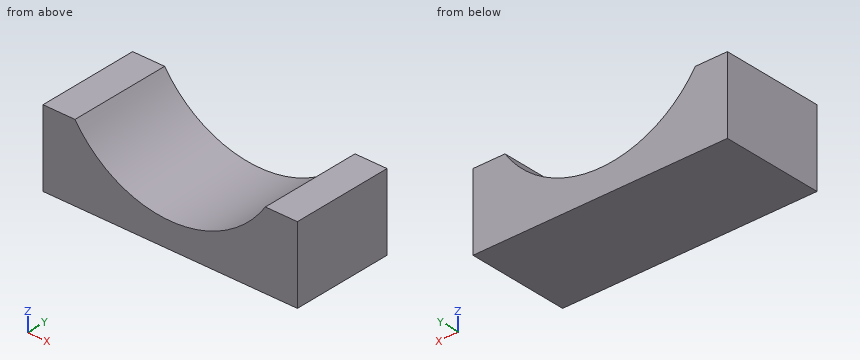
```python
from build123d import *

# Parameters (mm, degrees)
F0_W     = 50
F0_H     = 20
F1_DEPTH = 20
F2_R     = 22.5
F3_DEPTH = 25
F4_W     = 50
F4_H     = 5
F5_DEPTH = 25


with BuildPart() as f1:
    # F0 (on Top) → F1 (new body)
    with BuildSketch(Plane.XY):
        Rectangle(F0_W, F0_H)
    extrude(amount=F1_DEPTH)

    # F2 (on face) → F3 (cut)
    with BuildSketch(Plane.XZ.offset(10)):
        with Locations((0, 32.5)):
            Circle(F2_R)
    extrude(amount=-F3_DEPTH, mode=Mode.SUBTRACT)

    # F4 (on face) → F5 (cut)
    with BuildSketch(Plane.XZ.offset(10)):
        with Locations((0, 2.5)):
            Rectangle(F4_W, F4_H)
    extrude(amount=-F5_DEPTH, mode=Mode.SUBTRACT)


solid = f1.part
```
For this review, take the finished solid that the model builds, in its own axes (mm). Give positions to 0.01 mm unless a question says otherwise; leave off trailing zeros. Write each loop counter-clockwise with the first axis right and the second up, starting at its lowest first coordinate (ties: lowest second). Pieces come first, ordered by that corner, then holes.
Item 1: Wall thickness on probe 1 along X at (y, z) = (-5.5, 14.5); probe 2 along X at (y, z) = (0.75, 15.25); probe 3 along Z at (x, y) = (-1.5, -0.25): over which ranges is each line inside the solid? List them lowest first.
Item 2: Take a section at D-D (x = 17). Give the boundary of the cut face in (y, z), and give its area (3 significant figures).
Item 3: Take a section at B-B (y = 6.75). Give the boundary of the cut face in (x, z).
Item 4: Insertion check: P1, Ø6, axis at x = -2.5, y = -3, coming from the +Z side. The pin has a flat end and moves straight along its axis. Give the tip position at first contact, or say it passes through.
Item 5: Take a section at A-A (z = 14.5). Give the boundary of the cut face in (x, y), and give its area (3 significant figures).
Item 6: Take a section at C-C (z = 10.75). Give the boundary of the cut face in (x, y), and give its area (3 significant figures).
Established:
1. probe 1: x = -25 to -13.5, 13.5 to 25
1. probe 2: x = -25 to -14.45, 14.45 to 25
1. probe 3: z = 5 to 10.05
2. outline: (-10, 5) - (10, 5) - (10, 17.76) - (-10, 17.76) - close
2. area: 255 mm2
3. outline: (-25, 5) - (25, 5) - (25, 20) - (18.71, 20) arc R22.5 cw to (-18.71, 20) - (-25, 20) - close
4. P1: stops at z = 10.68
5. outline: (-25, -10) - (-13.5, -10) - (-13.5, 10) - (-25, 10) - close; (13.5, -10) - (25, -10) - (25, 10) - (13.5, 10) - close
5. area: 460 mm2
6. outline: (-25, -10) - (-5.76, -10) - (-5.76, 10) - (-25, 10) - close; (5.76, -10) - (25, -10) - (25, 10) - (5.76, 10) - close
6. area: 770 mm2
